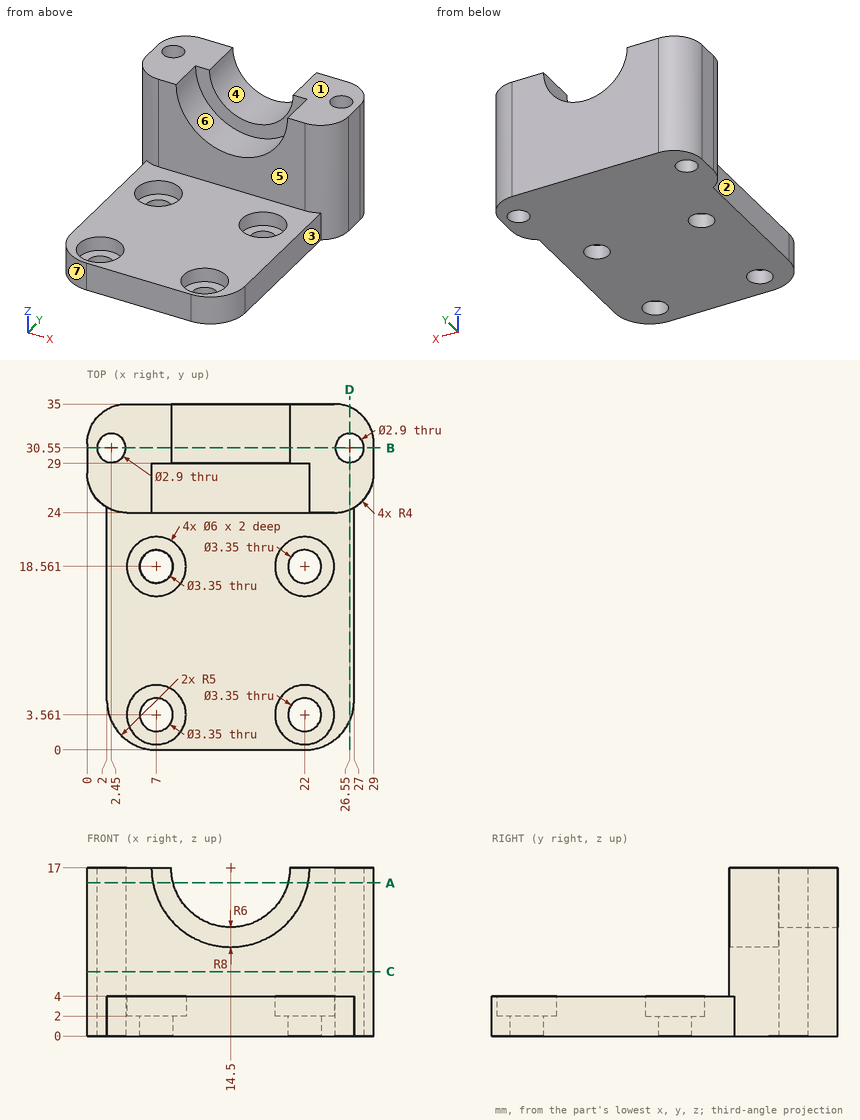
Check sheet for the drawn part. Datum: minimum x, y, z corner. Units: mm. A direction names the side the tool comes from. Round coordinates to 2 decimals unless told otherwise and drop trailing zeros. Loops run counter-clockwise (first coordinate to the right, second up) from the corner with the lowest first, then second, coordinate; pieces in that order, holes last. Notation, with made-up numbers: (50, -18.5) - (84, -18.5) arc R29 cw to (84, 9.5) - close; hole circle Ø1 at (-7, 84). An arc over 180 degrees is marked (long way). Answer as a JSON object with one key per item and string values. Group by question number.
Q1. Mould release check, pull along X, two halves, no side actions. Record for the marked faces 4, 5, 6 and 7: released by +X, released by -X, zero draft, split by the parting line, or undercut.
Q2. Sectioned sample at D-D, the plane x = 26.55. Enter the section's corners in (y, z).
Q3. Sectioned sample at A-A, the plane z = 15.5. Enter the section's corners in (x, y).
Q4. Scan lines: line 1 along Y through (x, z) = (22, 1.35) (1 decimal); line 2 along Y through (x, z) = (22, 2.7); line 3 along X through (y, z) = (30.5, 5.5). Record each from-to range of solid material in increasing order. Write a range as [from, to].
Q5. Set-up check for the marked faces 1, 2 and 3: record each of +Z, -Z, +X, -X, +Y, -Y from which the full face is reachable in a straight line by a thin tool's end or side.
Q6. Gauge pin test, flat ends, axial feed: P1, Ø1, axis at x = 15.5, y = 20.5, coming from the +Z side; P2, Ø4.5, axis at x = 7, y = 3.56, coming from the +Z side; P3, Ø2, axis at x = 22, y = 18.56, coming from the -Z side; P4, Ø1.2, axis at y = 17, z = 2.5, coming from the +X side. Record the tip position at first contact, or that the pin passes through.
Q7. Sectioned sample at C-C, the plane z = 6.5. Enter the section's corners in (x, y), plus the area to 3 significant figures.
Q8. Sectioned sample at B-B, the plane y = 30.55. Enter the section's corners in (x, z), plus the area to 3 significant figures.
Solution:
{
 "1": {"face 4": "undercut", "face 5": "zero draft", "face 6": "undercut", "face 7": "released by -X"},
 "2": {"outline": "(2.93, 0) - (29.1, 0) - (29.1, 17) - (24.31, 17) - (24.31, 4) - (2.93, 4) - close; (32, 0) - (34.69, 0) - (34.69, 17) - (32, 17) - close"},
 "3": {"outline": "(0, 28) arc R4 ccw to (4, 24) - (6.64, 24) - (6.64, 29) - (8.69, 29) - (8.69, 35) - (4, 35) arc R4 ccw to (0, 31) - close; (20.31, 29) - (22.36, 29) - (22.36, 24) - (25, 24) arc R4 ccw to (29, 28) - (29, 31) arc R4 ccw to (25, 35) - (20.31, 35) - close; hole circle Ø2.9 at (2.45, 30.55); hole circle Ø2.9 at (26.55, 30.55)"},
 "4": {"line 1": "y = [0, 1.9], [5.2, 16.9], [20.2, 35]", "line 2": "y = [0, 0.56], [6.56, 15.56], [21.56, 35]", "line 3": "x = [0, 1], [3.9, 25.1], [28, 29]"},
 "5": {"face 1": "+Z, +X, -X, +Y, -Y", "face 2": "+Z, -Z, -X, -Y", "face 3": "+Z, -Z, +X, -Y"},
 "6": {"P1": "stops at z = 4", "P2": "stops at z = 2", "P3": "passes through", "P4": "stops at x = 27"},
 "7": {"outline": "(0, 28) arc R4 ccw to (4, 24) - (25, 24) arc R4 ccw to (29, 28) - (29, 31) arc R4 ccw to (25, 35) - (4, 35) arc R4 ccw to (0, 31) - close; hole circle Ø2.9 at (2.45, 30.55); hole circle Ø2.9 at (26.55, 30.55)", "area": "292 mm²"},
 "8": {"outline": "(0, 0) - (1, 0) - (1, 17) - (0, 17) - close; (3.9, 0) - (25.1, 0) - (25.1, 17) - (20.5, 17) arc R6 cw to (8.5, 17) - (3.9, 17) - close; (28, 0) - (29, 0) - (29, 17) - (28, 17) - close", "area": "338 mm²"}
}
